The figure shows three views and two pictorial views of one solid part (mm, origin at its lowest corner). Answer the questions. A direction names the side the tool comes from. Round coordinates to 2 decimals unless told otherwise and drop trailing zeros. Write each loop counter-clockwise with the first axis right and the second up, starting at its lowest first coordinate (ties: lowest second). Pieces come first, ordered by that corner, then holes.
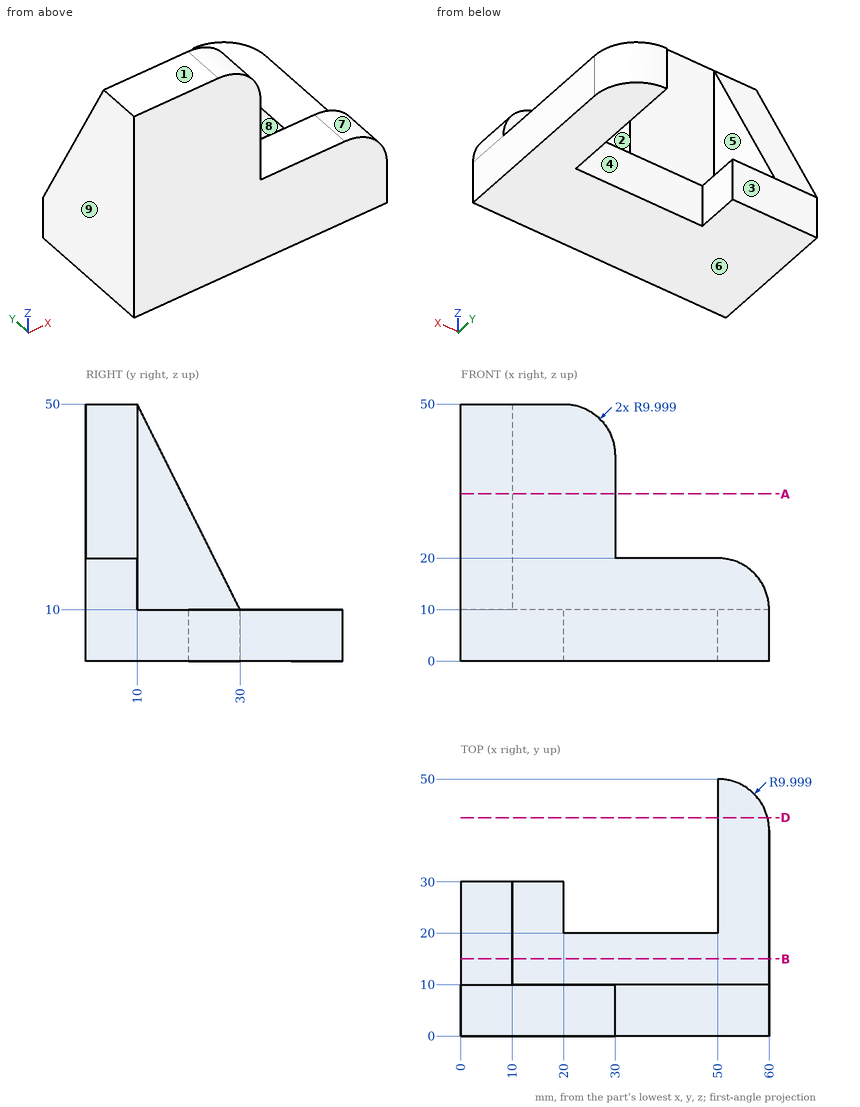
Q1. Determine the mould class of the marked faces 6, 7, 8 and 9 for opening direction X: pulls with the +X half, pulls with the -X half, needs draft (parallel to the pull), parting line crosses it, or undercut.
Verdict:
face 6: needs draft
face 7: pulls with the +X half
face 8: undercut
face 9: pulls with the -X half
Q2. Straight lines are drawn through the part: probe 1 along X at (y, z) = (6, 36.5); probe 2 along X at (y, z) = (34.5, 6); probe 3 along X at (y, z) = (24.5, 4). For each, find the intervals that lie inside material, in ascending order.
Verdict:
probe 1: x = 0 to 30
probe 2: x = 50 to 60
probe 3: x = 0 to 20, 50 to 60
Q3. Which of the six approach directions +Z, -Z, +X, -X, +Y, -Y give full straight-line access (tool end or side, diameter ignored) to the marked faces 1, 2, 3, 4 and 5?
Verdict:
face 1: +Z, +X, -X, +Y, -Y
face 2: +Z, +X, +Y, -Y
face 3: +Z, -Z, -X, +Y
face 4: +Z, -Z, +Y
face 5: +Z, +X, +Y
Q4. Section B-B (y = 15) is taken. Determine the outline of the cut face in (x, z), then the cut area to 3 significant figures.
Verdict:
outline: (0, 0) - (60, 0) - (60, 10) - (10, 10) - (10, 40) - (0, 40) - close
area: 900 mm2
Q5. Section A-A (z = 32.5) is taken. Determine the outline of the cut face in (x, y).
Verdict:
outline: (0, 0) - (30, 0) - (30, 10) - (10, 10) - (10, 18.75) - (0, 18.75) - close
Q6. Section D-D (y = 42.5) is taken. Determine the outline of the cut face in (x, z).
Verdict:
outline: (50, 0) - (59.68, 0) - (59.68, 10) - (50, 10) - close
Q7. Flat-ended cylindrical pins translate along their axes: pin 1 Ø8 at (y, z) = (41, 5.5) entering from -X; pin 2 Ø6 at (y, z) = (14, 44.5) entering from +X; pin 3 Ø3 at (y, z) = (3.5, 29) entering from +X. Find the tip coordinate at first contact, or state that the pin passes through.
Verdict:
pin 1: stops at x = 50
pin 2: stops at x = 10
pin 3: stops at x = 30
